Work out the finished part from the listing and answer in its coordinate system (mm). A direction names the side the tool comes from. Round coordinates to 2 decimals unless told otherwise and drop trailing zeros. Loops run counter-clockwise (first coordinate to the right, second up) from the corner with the lowest first, then second, coordinate; pieces in that order, holes last. Notation, with made-up numbers: (7, 85) - (37, 85) arc R30 cw to (37, 117) - close; hole circle Ø1 at (-9, 88.5). An arc over 180 degrees is marked (long way). Return JSON: item names as keys, results as strings.
from build123d import *

# Parameters (mm, degrees)
SKETCH1_W           = 20.34
SKETCH1_H           = 25.92
BOSS_EXTRUDE2_DEPTH = 6.93
SKETCH3_R           = 1.38
BOSS_EXTRUDE3_DEPTH = 3.158
SKETCH6_R           = 1.38
BOSS_EXTRUDE4_DEPTH = 3.158


with BuildPart() as part:
    # Sketch1 → Boss-Extrude2 (new body)
    with BuildSketch(Plane(origin=(0, 0, 0), x_dir=(1, 0, 0), z_dir=(0, 1, 0))):
        with Locations((10.17, -12.96)):
            Rectangle(SKETCH1_W, SKETCH1_H)
    extrude(amount=-BOSS_EXTRUDE2_DEPTH)

    # Sketch3 → Boss-Extrude3 (add)
    with BuildSketch(Plane(origin=(20.34, 0, 0), x_dir=(0, 0, -1), z_dir=(1, 0, 0))):
        with Locations(Location((-22.336733694, -3.465, 0), (0, 0, 180))):
            Circle(SKETCH3_R)
    extrude(amount=BOSS_EXTRUDE3_DEPTH)

    # Sketch6 → Boss-Extrude4 (add)
    with BuildSketch(Plane.ZY):
        with Locations(Location((21.694091509, -3.465, 0), (0, 0, 180))):
            Circle(SKETCH6_R)
    extrude(amount=BOSS_EXTRUDE4_DEPTH)


solid = part.part
1) A flat-ended cylindrical pin translates along its axis: pin 1 (3.5 mm diameter, centred on y = -2, z = 12, fed in from -X). Find the tip coordinate at first contact, or state that the pin passes through.
Verdict:
{"pin 1": "stops at x = 0"}
2) Section A-A (y = -0.5) is taken. Give the vertices of the cut face in (x, z), and give its area (3 significant figures).
Verdict:
{"outline": "(0, 0) - (20.34, 0) - (20.34, 25.92) - (0, 25.92) - close", "area": "527 mm2"}
3) Section C-C (x = 21) is taken. Give the vertices of the cut face in (y, z) (3 decimals), and give its area (3 significant figures).
Verdict:
{"outline": "circle Ø2.76 at (-3.465, 22.337)", "area": "5.98 mm2"}
4) Section B-B (z = 24.5) is taken. Give the vertices of the cut face in (x, y), and give its area (3 significant figures).
Verdict:
{"outline": "(0, -6.93) - (20.34, -6.93) - (20.34, 0) - (0, 0) - close", "area": "141 mm2"}
5) Find the intervals of material crossed by L1, parallel to X at y = -5, z = 8.25, in increasing order.
Verdict:
{"L1": "x = 0 to 20.34"}
6) Section D-D (y = -2.5) is taken. Give the vertices of the cut face in (x, z), and give its area (3 significant figures).
Verdict:
{"outline": "(-3.16, 20.71) - (0, 20.71) - (0, 0) - (20.34, 0) - (20.34, 21.35) - (23.5, 21.35) - (23.5, 23.32) - (20.34, 23.32) - (20.34, 25.92) - (0, 25.92) - (0, 22.68) - (-3.16, 22.68) - close", "area": "540 mm2"}
7) A tool of negligible diameter and unlimited length cuts with its end or side. For faces 1 (the flat face through (10, -3, 0)), 2 (the cylindrical face through (21.897, -3.88, 23.653)), 3 (the cylindrical face through (-1.56, -3.88, 20.38)), from which of +Z, -Z, +X, -X, +Y, -Y can it reach the whole face along a straight path? Write none if from no direction.
Verdict:
{"face 1": "-Z, +X, -X, +Y, -Y", "face 2": "+X", "face 3": "-X"}
